Input: part model. Units: mm. Frame: model coordinates. Give positions to 0.01 mm unless a question says otherwise; leave off trailing zeros. Loops run counter-clockwise (first coordinate to the right, second up) from the corner with the lowest first, then second, coordinate; pieces in that order, holes last. Notation, with made-up numbers: (-3.5, 65) -> (46.5, 65) arc R27 cw to (46.5, 86) -> close; hole circle Ø8 at (33, 15). An arc over 180 degrees is marked (long way). Answer in a Markdown table with one row per item. Add a question column.
```python
from build123d import *

# Parameters (mm, degrees)
F1_DEPTH  = 25
F1_FACE_W = 26.781376
F1_FACE_H = 25
F2_DEPTH  = 25
F3_R      = 4.013917
F4_DEPTH  = 25.001


with BuildPart() as f1:
    # F0 (on Top) → F1 (new body)
    with BuildSketch(Plane.XY):
        Polygon((-31.643473, 8.36918), (-58.424849, 44.396508), (-58.424849, 8.36918), align=None)
    extrude(amount=F1_DEPTH)

    # F1_face (on face) → F2 (join)
    with BuildSketch(Plane(origin=(-45.034161, 8.36918, 12.5), x_dir=(1, 0, 0), z_dir=(0, -1, 0))):
        Rectangle(F1_FACE_W, F1_FACE_H)
    extrude(amount=F2_DEPTH)

    # F3 (on face) → F4 (cut, through all)
    with BuildSketch(Plane(origin=(0, 0, 0), x_dir=(1, 0, 0), z_dir=(0, 0, -1))):
        with Locations((-51.251266, -21.759868)):
            Circle(F3_R)
    extrude(amount=-F4_DEPTH, mode=Mode.SUBTRACT)


solid = f1.part
```
1) Pull-direction query (Y, two-part tool) for faces 1 (the face through (-44.847, 26.131, 12.325)), 2 (the face through (-48, 8, 25)), 3 (the face through (-45, -16.631, 13)), 4 (the face through (-49.4, 25.32, 12.32)); classes: +Y half, -Y half, draft (parallel to the pull), parting line (faces both ways), or undercut.
2) Section C-C on z = 16.5. Output: boundary loops of the cut face in (x, y), and give its area (3 significant figures).
3) Section A-A on x = -53.5. Output: boundary loops of the cut face in (y, z) (3 decimals).
4) Material intervals for line 1 along Y through (x, z) = (-54.75, 1.75); line 2 along X through (y, z) = (24.5, 11.75); line 3 along X through (y, z) = (35.5, 3.5), sorted ascending.
5) Section B-B on y = 21. Output: boundary loops of the cut face in (x, z).
6) Section D-D on y = 31. Output: boundary loops of the cut face in (x, z).
7) Pin query (flat end, axial travel): pin 1 (1.5 mm diameter, centred on x = -37.5, z = 21.5, fed in from +Y); pin 2 (4 mm diameter, centred on x = -48, y = 6.5, fed in from -Z). Return the tip coordinate at first contact, or that it passes through.
Working result:
| question | item | result |
|---|---|---|
| 1 | face 1 | +Y half |
| 1 | face 2 | draft |
| 1 | face 3 | -Y half |
| 1 | face 4 | undercut |
| 2 | outline | (-58.42, -16.63) -> (-31.64, -16.63) -> (-31.64, 8.37) -> (-58.42, 44.4) -> close; hole circle Ø8.03 at (-51.25, 21.76) |
| 2 | area | 1,100 mm2 |
| 3 | outline | (-16.631, 0) -> (18.435, 0) -> (18.435, 25) -> (-16.631, 25) -> close; (25.085, 0) -> (37.771, 0) -> (37.771, 25) -> (25.085, 25) -> close |
| 4 | line 1 | y = -16.63 to 19.79, 23.73 to 39.45 |
| 4 | line 2 | x = -58.42 to -54.18, -48.32 to -43.63 |
| 4 | line 3 | x = -58.42 to -51.81 |
| 5 | outline | (-58.42, 0) -> (-55.19, 0) -> (-55.19, 25) -> (-58.42, 25) -> close; (-47.31, 0) -> (-41.03, 0) -> (-41.03, 25) -> (-47.31, 25) -> close |
| 6 | outline | (-58.42, 0) -> (-48.47, 0) -> (-48.47, 25) -> (-58.42, 25) -> close |
| 7 | pin 1 | stops at y = 17.26 |
| 7 | pin 2 | stops at z = 0 |
